```python
from build123d import *

# Parameters (mm, degrees)
BOSS_EXTRUDE1_DEPTH      = 10
BOSS_EXTRUDE1_DEPTH_BACK = 10
SKETCH1_R                = 6.825
CUT_EXTRUDE1_DEPTH       = 14.898246292
CUT_EXTRUDE1_DEPTH_BACK  = 14.898246292
SKETCH2_R                = 2.6
FILLET1_R                = 1
FILLET2_R                = 0.5


with BuildPart() as part:
    # Sketch1 → Boss-Extrude1 (new, two sides: drawn at the far end of the back side and taken through both)
    with BuildSketch(Plane.XY.offset(-BOSS_EXTRUDE1_DEPTH_BACK)):
        Circle(SKETCH1_R)
    extrude(amount=BOSS_EXTRUDE1_DEPTH + BOSS_EXTRUDE1_DEPTH_BACK)

    # Sketch2 → Cut-Extrude1 (cut, two sides: drawn at the far end of the back side and taken through both)
    with BuildSketch(Plane(origin=(0, 0, 0), x_dir=(1, 0, 0), z_dir=(0, 1, 0)).offset(-CUT_EXTRUDE1_DEPTH_BACK)):
        with Locations(Location((0, 0, 0), (0, 0, 270))):
            Circle(SKETCH2_R)
    extrude(amount=CUT_EXTRUDE1_DEPTH + CUT_EXTRUDE1_DEPTH_BACK, mode=Mode.SUBTRACT)

    # Fillet1
    fillet1_edges = [part.edges().sort_by_distance(p)[0] for p in [
        (-6.825, 0, 10),
        (-6.825, 0, -10),
    ]]
    fillet(fillet1_edges, radius=FILLET1_R)

    # Fillet2
    fillet2_edges = [part.edges().sort_by_distance(p)[0] for p in [
        (0, -6.825, -2.600000002),
        (1e-09, 6.825, -2.600000001),
    ]]
    fillet(fillet2_edges, radius=FILLET2_R)


solid = part.part
```
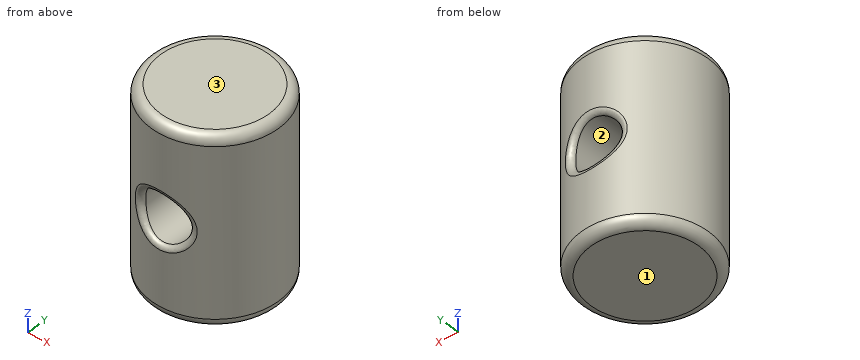
Geometry: final body of the model. Coordinates: model frame, mm. Face numbers are marked on the shaded views. Give positions to 0.01 mm unless a question says otherwise; leave off trailing zeros. Write each loop counter-clockwise with the first axis right and the second up, starting at its lowest first coordinate (ties: lowest second). Pieces come first, ordered by that corner, then holes.
1. Section query A-A, the plane y = 0. Return loops of the section in (x, z) (3 decimals).
2. Draft query along Z for the marked faces 1, 2 and 3. Return one class per face: released by +Z, released by -Z, zero draft, split by the parting line, or undercut.
3. Pin query (flat end, axial travel): P1, Ø4, axis at y = 4, z = 3.5, coming from the +X side; P2, Ø3, axis at x = 3.5, z = -6, coming from the -Y side; P3, Ø1.5, axis at x = 1, z = -2, coming from the +Y side. Return the tip coordinate at first contact, or that it passes through.
4. Line query: probe 1 along Z at (x, y) = (0, -2); probe 2 along Z at (x, y) = (1.5, 3); probe 3 along Y at (x, z) = (-0.25, -3.25). Output: solid intervals per line, ascending.
5. Section query B-B, the plane z = -6.75. Return loops of the section in (x, y) (3 decimals).
Computed:
1. outline: (-6.825, -9) arc R1 ccw to (-5.825, -10) - (5.825, -10) arc R1 ccw to (6.825, -9) - (6.825, 9) arc R1 ccw to (5.825, 10) - (-5.825, 10) arc R1 ccw to (-6.825, 9) - close; hole circle Ø5.2 at (0, 0)
2. face 1: released by -Z
2. face 2: undercut
2. face 3: released by +Z
3. P1: stops at x = 6.53
3. P2: stops at y = -6.53
3. P3: stops at y = 6.71
4. probe 1: z = -10 to -2.6, 2.6 to 10
4. probe 2: z = -10 to -2.12, 2.12 to 10
4. probe 3: y = -6.82 to 6.82
5. outline: circle Ø13.65 at (0, 0)
